The model under review builds one solid part; all positions refer to its coordinate system, in mm. A direction names the side the tool comes from. Round coordinates to 2 decimals unless told otherwise and drop trailing zeros. Write each loop counter-clockwise with the first axis right and the second up, starting at its lowest first coordinate (ties: lowest second). Pieces come first, ordered by that corner, then holes.
Item 1: Machinability: for faces 5 (the face through (0, 3, 1.05)), 6 (the face through (13, 3, 14)), which of the approach directions +Z, -Z, +X, -X, +Y, -Y give a long, thin tool a straight path to every point of the face, cutting with its end or side? Answer none if there is none.
Item 2: Add section A-A (x = 0). Give the boundary of the cut face in (y, z) (3 decimals), plus the area to 3 significant figures.
Item 3: Draft analysis for pull direction Z (two halves, no side actions). For faces 1 (the face through (-15, 3, 0)), 2 (the face through (-9.544, 2.958, 8.809)), 3 (the face through (-14, 3, 13)), 4 (the face through (13, 3, -14)), state which applies: +Z half, -Z half, draft (parallel to the pull), parting line (faces both ways), or undercut.
Item 4: Clearance check with a flat-ended pin moving along its axis: pin 1 Ø7 at (x, z) = (7.53, -7.05) entering from -Y. State where the tip first meets the part, or that it passes through.
Item 5: To check wall thickness, follow L1, parallel to X at y = 5.2, z = -7.75; L2, parallel to X at y = 0.9, z = -8; L3, parallel to X at y = 3.7, z = 0 (3 decimals). State the ranges of each line that lie inside material, in increasing order.
Item 6: Add section C-C (y = 4.05). State how many separate pieces and enclosed holes the cut face has, plus the area to 3 significant figures.
Item 7: Add section B-B (z = 0). Give the boundary of the cut face in (x, y) (3 decimals).
Item 8: Add section D-D (x = 6.5). Give the boundary of the cut face in (y, z), plus the area to 3 significant figures.
```python
from build123d import *

# Parameters (mm, degrees)
SKETCH1_W             = 30
SKETCH1_H             = 30
BOSS_EXTRUDE1_DEPTH   = 6
FILLET1_R             = 5
F_8_CLEARANCE_HOLE1_D = 4.4958


with BuildPart() as part:
    # Sketch1 → Boss-Extrude1 (new body)
    with BuildSketch(Plane(origin=(0, 0, 0), x_dir=(1, 0, 0), z_dir=(0, 1, 0))):
        Rectangle(SKETCH1_W, SKETCH1_H)
        with BuildLine():
            Line((1.731509457, -1.05), (-1.731509457, -1.05))
            ThreePointArc((-1.731509457, -1.05), (0, 2.025), (1.731509457, -1.05))
        make_face(mode=Mode.SUBTRACT)
    extrude(amount=BOSS_EXTRUDE1_DEPTH)

    # Fillet1
    fillet1_edges = [part.edges().sort_by_distance(p)[0] for p in [
        (15, 3, 15),
        (-15, 3, 15),
        (-15, 3, -15),
        (15, 3, -15),
    ]]
    fillet(fillet1_edges, radius=FILLET1_R)

    # #8 Clearance Hole1 (through all)
    with Locations(Plane(origin=(0, 6, 0), x_dir=(1, 0, 0), z_dir=(0, 1, 0))):
        with Locations((-7.467684416, 7.05158171), (7.532315584, 7.05158171), (-7.467684416, -7.94841829), (7.532315584, -7.94841829)):
            Hole(F_8_CLEARANCE_HOLE1_D / 2)


solid = part.part
```
Numbers:
1. face 5: +Y, -Y
1. face 6: +Z, +X, +Y, -Y
2. outline: (0, -15) - (6, -15) - (6, -2.025) - (0, -2.025) - close; (0, 1.05) - (6, 1.05) - (6, 15) - (0, 15) - close
2. area: 162 mm2
3. face 1: draft
3. face 2: undercut
3. face 3: +Z half
3. face 4: -Z half
4. pin 1: stops at y = 0
5. L1: x = -15 to -9.6, -5.33 to 5.4, 9.67 to 15
5. L2: x = -15 to -9.51, -5.43 to 5.49, 9.57 to 15
5. L3: x = -15 to -2.025, 2.025 to 15
6. separate pieces: 1
6. enclosed holes: 5
6. area: 805 mm2
7. outline: (-15, 0) - (-2.025, 0) - (-2.025, 6) - (-15, 6) - close; (2.025, 0) - (15, 0) - (15, 6) - (2.025, 6) - close
8. outline: (0, -15) - (6, -15) - (6, -9.05) - (0, -9.05) - close; (0, -5.05) - (6, -5.05) - (6, 5.95) - (0, 5.95) - close; (0, 9.95) - (6, 9.95) - (6, 15) - (0, 15) - close
8. area: 132 mm2
